Input: part model. Units: mm. Frame: model coordinates. A direction names the side the tool comes from. Coordinates: 2 decimals unless noted, no trailing zeros. Order: outer loops, then holes, each group sorted by start corner. A loop starts at its lowest first (then second) coordinate and runs counter-clockwise, first axis right, second up. Notation, with made-up numbers: (23, 3) -> (46, 3) arc R10 ccw to (46, 11) -> close; hole circle Ø10 at (-33, 46). An arc over 180 degrees is marked (long way). One line per question, with ' | ' between items.
```python
from build123d import *

# Parameters (mm, degrees)
MAIN_DEPTH                = 120
PERNO1_START              = 160
PERNO1_OUTLINE_R          = 51.5
PERNO1_DEPTH              = 94
PERNO1_2_OUTLINE_R        = 65
PERNO1_2_DEPTH            = 120
SANALATURAPERNO_START     = 254
SKETCH4_3_R               = 40
SANALATURAPERNO_DEPTH     = 5
PERNO2_START              = 259
SKETCH4_4_R               = 51.5
SKETCH4_4_R_2             = 40
PERNO2_DEPTH              = 10
CHAMFER1_SIZE             = 4
FILLET2_R                 = 8
CHAMFER1_OF_MIRROR14_SIZE = 4
FILLET2_OF_MIRROR14_R     = 8
CHAMFER2_SIZE             = 5
PISTA_R                   = 17
SKETCH9_W                 = 397.156797082
SKETCH9_H                 = 271.545663618
CUT_EXTRUDE4_DEPTH        = 120
FILLET3_R                 = 0.5


# Read off the part's stored shape, not the designer's step: Perno1
with BuildPart() as part:
    # MainBody → Main (new body)
    with BuildSketch(Plane(origin=(0, 0, 0), x_dir=(1, 0, 0), z_dir=(0, 1, 0))):
        Polygon((-110, 160), (110, 160), (170, 100), (170, -100), (110, -160), (-110, -160), (-170, -100), (-170, 100), align=None)
    extrude(amount=MAIN_DEPTH)

    # Perno1 outline → Perno1 (add)
    with BuildSketch(Plane.XY.offset(PERNO1_START)):
        with Locations((0, 60)):
            Circle(PERNO1_OUTLINE_R)
    perno1 = extrude(amount=PERNO1_DEPTH)

    # Perno1 2 outline → Perno1 2 (cut)
    with BuildSketch(Plane(origin=(0, 0, 0), x_dir=(1, 0, 0), z_dir=(0, 1, 0))):
        Circle(PERNO1_2_OUTLINE_R)
    perno1_2 = extrude(amount=PERNO1_2_DEPTH, mode=Mode.SUBTRACT)

    # Sketch4<3> → SanalaturaPerno (add)
    with BuildSketch(Plane.XY.offset(SANALATURAPERNO_START)):
        with Locations(Location((0, 60, 0), (0, 0, 180))):
            Circle(SKETCH4_3_R)
    sanalaturaperno = extrude(amount=SANALATURAPERNO_DEPTH)

    # Sketch4<4> → Perno2 (add)
    # profile 1 of 2: a face of its own
    with BuildSketch(Plane.XY.offset(PERNO2_START)):
        with Locations(Location((0, 60, 0), (0, 0, 180))):
            Circle(SKETCH4_4_R)
        with Locations(Location((0, 60, 0), (0, 0, 180))):
            Circle(SKETCH4_4_R_2, mode=Mode.SUBTRACT)
    # profile 2 of 2: a face of its own
    with BuildSketch(Plane.XY.offset(PERNO2_START)):
        with Locations(Location((0, 60, 0), (0, 0, 180))):
            Circle(SKETCH4_4_R_2)
    perno2 = extrude(amount=PERNO2_DEPTH)

    # Chamfer1
    chamfer1_edges = [part.edges().sort_by_distance(p)[0] for p in [
        (51.5, 60, 269),
    ]]
    chamfer(chamfer1_edges, length=CHAMFER1_SIZE)

    # Fillet2
    fillet2_edges = [part.edges().sort_by_distance(p)[0] for p in [
        (-51.5, 60, 160),
    ]]
    fillet(fillet2_edges, radius=FILLET2_R)

    # Mirror14: Perno1, Perno1 2, SanalaturaPerno, Perno2 across plane
    add(perno1.mirror(Plane.XY))
    add(perno1_2.mirror(Plane.XY), mode=Mode.SUBTRACT)
    add(sanalaturaperno.mirror(Plane.XY))
    add(perno2.mirror(Plane.XY))

    # Chamfer1 of Mirror14
    chamfer1_of_mirror14_edges = [part.edges().sort_by_distance(p)[0] for p in [
        (51.5, 60, -269),
    ]]
    chamfer(chamfer1_of_mirror14_edges, length=CHAMFER1_OF_MIRROR14_SIZE)

    # Fillet2 of Mirror14
    fillet2_of_mirror14_edges = [part.edges().sort_by_distance(p)[0] for p in [
        (-51.5, 60, -160),
    ]]
    fillet(fillet2_of_mirror14_edges, radius=FILLET2_OF_MIRROR14_R)

    # Chamfer2
    chamfer2_edges = [part.edges().sort_by_distance(p)[0] for p in [
        (-65, 0, 0),
    ]]
    chamfer(chamfer2_edges, length=CHAMFER2_SIZE)

    # Pista → PistaCut (revolve, cut)
    with BuildSketch(Plane.XY, mode=Mode.PRIVATE) as pistacut_sk:
        with Locations((106, 128)):
            Circle(PISTA_R)
    revolve(pistacut_sk.sketch.rotate(Axis((0, 120, 0), (0, -1, 0)), 90), axis=Axis((0, 120, 0), (0, -1, 0)), mode=Mode.SUBTRACT)

    # Sketch8 → Cut-Revolve2 (revolve, cut)
    with BuildSketch(Plane(origin=(0, 0, 0), x_dir=(0, 0, -1), z_dir=(1, 0, 0))):
        Polygon((-136, 141), (-136, 131), (-136, 120), (-136, 110), (-130, 110), (-130, 120), (-130, 124), (-130, 141), align=None)
    revolve(axis=Axis((0, 120, 0), (0, -1, 0)), mode=Mode.SUBTRACT)

    # Sketch9 → Cut-Extrude4 (cut)
    with BuildSketch(Plane(origin=(0, 0, 0), x_dir=(1, 0, 0), z_dir=(0, 1, 0))):
        with Locations((-21.107680821, 135.772831809)):
            Rectangle(SKETCH9_W, SKETCH9_H)
    extrude(amount=CUT_EXTRUDE4_DEPTH, mode=Mode.SUBTRACT)

    # Fillet3
    fillet3_edges = [part.edges().sort_by_distance(p)[0] for p in [
        (0, 110, 136),
        (0, 110, 136),
        (0, 110, 130),
        (0, 110, 130),
        (0, 110, 130),
        (0, 110, 136),
    ]]
    fillet(fillet3_edges, radius=FILLET3_R)


solid = part.part
```
1. Ray query, line 1 (Z direction, x = -40, y = 67); line 2 (Z direction, x = 19.5, y = 23.5); line 3 (Z direction, x = -100, y = 13.5). Return the intervals inside material, ascending. Write a range as [from, to].
Recorded:
line 1: z = [51.23, 254], [259, 269] | line 2: z = [62.01, 254], [259, 269] | line 3: z = [0, 160]
2. Access query for faces 1 (the face through (2.991, 115.184, 135.967)), 2 (the face through (-1.429, 61.695, 64.984)), 3 (the face through (26.5, 29.7, 254)), 4 (the face through (27.686, 103.425, 210.398)). Directions: +Z, -Z, +X, -X, +Y, -Y. A direction counts if a zero-diameter tool reaches every point of the face in a straight line with its end or side. Return the directions, or none.
Recorded:
face 1: +Y | face 2: -Z, +Y, -Y | face 3: none | face 4: +Z
3. Pin query (flat end, axial travel): pin 1 Ø4 at (x, z) = (-6.5, 115) entering from +Y; pin 2 Ø5 at (x, y) = (-18.5, 13) entering from -Z; pin 3 Ø4 at (x, y) = (75.5, 19.5) entering from +Z. Return the tip coordinate at first contact, or that it passes through.
Recorded:
pin 1: stops at y = 115.2 | pin 2: stops at z = 61.51 | pin 3: stops at z = 160
4. Cut plane B-B, the plane y = 60. Return loops of the section in (x, z), and give its area (3 significant figures).
Recorded:
outline: (-170, 0) -> (-65, 0) arc R65 cw to (65, 0) -> (170, 0) -> (170, 100) -> (110, 160) -> (59.5, 160) arc R8 cw to (51.5, 168) -> (51.5, 254) -> (40, 254) -> (40, 259) -> (51.5, 259) -> (51.5, 265) -> (47.5, 269) -> (-47.5, 269) -> (-51.5, 265) -> (-51.5, 259) -> (-40, 259) -> (-40, 254) -> (-51.5, 254) -> (-51.5, 168) arc R8 cw to (-59.5, 160) -> (-110, 160) -> (-170, 100) -> close | area: 55,300 mm^2
5. Cut plane C-C, the plane z = 175.5. Return loops of the section in (x, y).
Recorded:
outline: circle Ø103 at (0, 60)
6. Mould query, pull axis X, two halves, no side actions, for faces 5 (the face through (-11, 110, 133)), 6 (the face through (170, 59, 49)), 7 (the face through (1, 120, 122)). Classes: released by +X, released by -X, zero draft, split by the parting line, or undercut.
Recorded:
face 5: undercut | face 6: released by +X | face 7: zero draft
